```python
from build123d import *

# Parameters (mm, degrees)
BOSS_EXTRUDE1_DEPTH = 200
CHAMFER1_SIZE       = 3
SKETCH2_W           = 5
SKETCH2_H           = 4.1
CUT_EXTRUDE1_DEPTH  = 200
LPATTERN1_COUNT     = 20
LPATTERN1_PITCH     = 10
BOSS_EXTRUDE2_DEPTH = 25
CHAMFER2_SIZE       = 4


with BuildPart() as part:
    # Sketch1 → Boss-Extrude1 (new body)
    with BuildSketch(Plane.XY):
        Polygon((-14, 2.3), (-7.8, 2.3), (-7.8, 4.9), (-10.5, 7.6), (-6.4, 11.7), (6.4, 11.7), (10.5, 7.6), (7.8, 4.9), (7.8, 2.3), (14, 2.3), (14, -4.7), (10, -4.7), (10, -0.7), (-10, -0.7), (-10, -4.7), (-14, -4.7), align=None)
    extrude(amount=BOSS_EXTRUDE1_DEPTH)

    # Chamfer1
    chamfer1_edges = [part.edges().sort_by_distance(p)[0] for p in [
        (-14, 2.3, 100),
        (14, 2.3, 100),
    ]]
    chamfer(chamfer1_edges, length=CHAMFER1_SIZE)

    # Sketch2 → Cut-Extrude1 (cut, symmetric)
    with BuildSketch(Plane(origin=(0, 0, 0), x_dir=(0, 0, -1), z_dir=(1, 0, 0))):
        with Locations((-192.5, 9.65)):
            Rectangle(SKETCH2_W, SKETCH2_H)
    cut_extrude1 = extrude(amount=CUT_EXTRUDE1_DEPTH, both=True, mode=Mode.SUBTRACT)

    # LPattern1: Cut-Extrude1 ×20
    with Locations(*[(0, 0, -i * LPATTERN1_PITCH) for i in range(1, LPATTERN1_COUNT)]):
        add(cut_extrude1, mode=Mode.SUBTRACT)

    # Sketch4 → Boss-Extrude2 (add)
    with BuildSketch(Plane(origin=(0, 0, 25), x_dir=(-1, 0, 0), z_dir=(0, 0, -1))):
        Polygon((-10.5, 7.6), (10.5, 7.6), (6.4, 11.7), (-6.4, 11.7), align=None)
    extrude(amount=BOSS_EXTRUDE2_DEPTH)

    # Chamfer2
    chamfer2_edges = [part.edges().sort_by_distance(p)[0] for p in [
        (0, 11.7, 0),
    ]]
    chamfer(chamfer2_edges, length=CHAMFER2_SIZE)


solid = part.part
```
Geometry check sheet. Reference: the model listing, model coordinates, mm. A direction names the side the tool comes from. Coordinates: 2 decimals unless noted, no trailing zeros. Order: outer loops, then holes, each group sorted by start corner. A loop starts at its lowest first (then second) coordinate and runs counter-clockwise, first axis right, second up. Notation, with made-up numbers: M -35,10.25 L -16,10.25 A35 ccw -16,48.25 Z; hole C -7.5,-19 d2. An arc over 180 degrees is marked long. Answer as a JSON object with one key per item and string values.
Q1. Cross-section at A-A on y = -2.5. Record the cut outline in (x, z).
Results are:
{"outline": "M -14,0 L -10,0 L -10,200 L -14,200 Z; M 10,0 L 14,0 L 14,200 L 10,200 Z"}
Q2. Tool access check on faces 1 (the flat face through (0, -0.7, 99)), 2 (the flat face through (9, 2.3, 99)), 3 (the flat face through (8.4, 9.7, 57.5)), 4 (the flat face through (-8.5, 9.6, 127.5)), 5 (the flat face through (0, 10, 180)). Record the directions out of +Z, -Z, +X, -X, +Y, -Y that give a thin tool (end or side, any length) a straight path to the whole face; none if there is none.
Results are:
{"face 1": "+Z, -Z, -Y", "face 2": "+Z, -Z, +X", "face 3": "+Z, -Z, +X, +Y", "face 4": "+Z, -Z, -X, +Y", "face 5": "+X, -X, +Y"}
Q3. Scan lines: line 1 (X direction, y = -2, z = 46); line 2 (Y direction, x = -1.25, z = 28.5); line 3 (Y direction, x = 3.5, z = 93). Record each from-to range of solid material in increasing order.
Results are:
{"line 1": "x = -14 to -10, 10 to 14", "line 2": "y = -0.7 to 11.7", "line 3": "y = -0.7 to 7.6"}
Q4. Cross-section at B-B on z = 92. Record the cut outline in (x, y), and give its area (3 significant figures).
Results are:
{"outline": "M -14,-4.7 L -10,-4.7 L -10,-0.7 L 10,-0.7 L 10,-4.7 L 14,-4.7 L 14,-0.7 L 11,2.3 L 7.8,2.3 L 7.8,4.9 L 10.5,7.6 L -10.5,7.6 L -7.8,4.9 L -7.8,2.3 L -11,2.3 L -14,-0.7 Z", "area": "197 mm²"}
Q5. Release check for a two-part mould opening along Z. For faces 6 (the flat face through (8.4, 9.7, 137.5)), 7 (the flat face through (0, 10, 160)) record: released by +Z, released by -Z, zero draft, split by the parting line, or undercut.
Results are:
{"face 6": "zero draft", "face 7": "undercut"}
Q6. Depth check by flat-ended pin: pin 1 Ø2 at (x, y) = (-3, 9) entering from -Z; pin 2 Ø5 at (x, z) = (9.5, 122) entering from +Y; pin 3 Ø4 at (x, z) = (-4.5, 60) entering from -Y. Enter the tip coordinate at first touch or a pass-through.
Results are:
{"pin 1": "stops at z = 0.3", "pin 2": "stops at y = 10.1", "pin 3": "stops at y = -0.7"}
